The model under review builds one solid part; all positions refer to its coordinate system, in mm. A direction names the side the tool comes from. Round coordinates to 2 decimals unless told otherwise and drop trailing zeros. Write each loop counter-clockwise with the first axis right and the second up, starting at its lowest first coordinate (ties: lowest second). Pieces come first, ordered by that corner, then holes. Notation, with made-up numbers: M 54.5,51.25 L 80.5,51.25 A12 cw 80.5,59.25 Z; hole C 2.5,-26.5 d11. An arc over 180 degrees is marked long. One line per item, written item: value. Start each with the question number.
1) Tool access review of faces 1 (the face through (1, 5, 26.5)), 2 (the face through (-100, 5, 26.5)), 3 (the face through (99.29, -6.52, 3.19)), 4 (the face through (-22, 8, -13.95)): name each direction out of +Z, -Z, +X, -X, +Y, -Y from which nothing blocks a thin tool from reaching the whole face with its end or side.
2) Mouldability with a two-part tool opening along X and no side actions: class faces 5 (the face through (-31, 10, 13)), 6 (the face through (-113.57, 4.93, 25)), 7 (the face through (-41, 3, -21.227)) as +X half, -X half, draft (parallel to the pull), parting line (faces both ways), or undercut.
3) Wall thickness on probe 1 along Z at (x, y) = (75, 8.2); probe 2 along Z at (x, y) = (-12.5, 1.5); probe 3 along X at (y, z) = (5, 20.5): over which ranges is each line inside the solid? List them lowest first.
4) Take a section at B-B, the plane x = 75. Write out the cut boundary in (y, z).
5) Take a section at A-A, the plane x = -5. Write out the cut boundary in (y, z).
6) For P1, Ø1.8, axis at x = -50.5, y = 2.5, coming from the +Z side; P2, Ø8, axis at y = -5, z = 16.5, coming from the -X side; P3, Ø3, axis at x = -52.5, y = 7.5, coming from the -Z side; P4, Ø1.5, axis at x = -71.5, y = -1, coming from the -Z side, all flat-tipped, find the tip position at first contact; note any pin that passes through.
from build123d import *

# Parameters (mm, degrees)
BOSS_EXTRUDE1_DEPTH     = 10
SKETCH2_W               = 50
SKETCH2_H               = 42.5
CUT_EXTRUDE1_DEPTH      = 6
CUT_EXTRUDE7_REACH      = 111.659
SKETCH10_R              = 14.5
CUT_EXTRUDE8_DEPTH      = 110.658560997
CUT_EXTRUDE8_DEPTH_BACK = 3
SKETCH11_R              = 18.75
BOSS_EXTRUDE3_START     = 8
SKETCH12_R              = 30
BOSS_EXTRUDE3_DEPTH     = 8
SKETCH13_R              = 24.5
CUT_EXTRUDE9_DEPTH      = 3
SKETCH14_R              = 18.75
CUT_EXTRUDE10_DEPTH     = 7
CUT_EXTRUDE11_START     = -6
SKETCH15_R              = 24.5
CUT_EXTRUDE11_DEPTH     = 6
CUT_EXTRUDE19_REACH     = 112.095
SKETCH26_W              = 40
SKETCH26_H              = 53
BOSS_EXTRUDE5_DEPTH     = 10
SKETCH19_W              = 46.483409888
SKETCH19_H              = 53
BOSS_EXTRUDE4_DEPTH     = 10
SKETCH23_W              = 7
SKETCH23_H              = 42.47741106
CUT_EXTRUDE18_DEPTH     = 6
FILLET3_R               = 5
SKETCH27_R              = 2.05
SKETCH27_R_2            = 4.962590862
CUT_EXTRUDE20_DEPTH     = 20
CUT_EXTRUDE22_REACH     = 121.269
SKETCH29_R              = 2.05
CUT_EXTRUDE23_REACH     = 121.269
SKETCH30_R              = 1.25


with BuildPart() as part:
    # Sketch1 → Boss-Extrude1 (new body)
    with BuildSketch(Plane(origin=(0, 0, 0), x_dir=(1, 0, 0), z_dir=(0, 1, 0))):
        with BuildLine():
            Line((-52.13627327, 26.5), (60.93763889, 26.5))
            ThreePointArc((60.93763889, 26.5), (105, 0), (60.93763889, -26.5))
            Line((60.93763889, -26.5), (-52.13627327, -26.5))
            Line((-52.13627327, -26.5), (-60.93763889, -26.5))
            ThreePointArc((-60.93763889, -26.5), (-105, 0), (-60.93763889, 26.5))
            Line((-60.93763889, 26.5), (-52.13627327, 26.5))
        make_face()
    extrude(amount=BOSS_EXTRUDE1_DEPTH)

    # Sketch2 → Cut-Extrude1 (cut)
    with BuildSketch(Plane.XZ):
        with Locations((-37.25, 0.02258894)):
            Rectangle(SKETCH2_W, SKETCH2_H)
    extrude(amount=-CUT_EXTRUDE1_DEPTH, mode=Mode.SUBTRACT)

    # Sketch10 → Cut-Extrude7 (cut, up to next)
    with BuildSketch(Plane.XZ, mode=Mode.PRIVATE) as cut_extrude7_sk1:
        with Locations(Location((75, 0, 0), (0, 0, 270))):
            Circle(SKETCH10_R)
    cut_extrude7_tool1 = extrude(cut_extrude7_sk1.sketch, amount=-CUT_EXTRUDE7_REACH, mode=Mode.PRIVATE) & part.part
    add(cut_extrude7_tool1.solids().sort_by_distance((75, 0, 0))[0], mode=Mode.SUBTRACT)

    # Sketch11 → Cut-Extrude8 (cut, two sides: drawn at the far end of the back side and taken through both)
    with BuildSketch(Plane.XZ.offset(-CUT_EXTRUDE8_DEPTH_BACK)):
        with Locations(Location((75, 0, 0), (0, 0, 90))):
            Circle(SKETCH11_R)
    extrude(amount=CUT_EXTRUDE8_DEPTH + CUT_EXTRUDE8_DEPTH_BACK, mode=Mode.SUBTRACT)

    # Sketch12 → Boss-Extrude3 (add)
    with BuildSketch(Plane.XZ.offset(BOSS_EXTRUDE3_START)):
        with Locations(Location((75, 0, 0), (0, 0, 270))):
            Circle(SKETCH12_R)
    extrude(amount=-BOSS_EXTRUDE3_DEPTH)

    # Sketch13 → Cut-Extrude9 (cut)
    with BuildSketch(Plane.XZ.offset(8)):
        with Locations(Location((75, 0, 0), (0, 0, 270))):
            Circle(SKETCH13_R)
    extrude(amount=-CUT_EXTRUDE9_DEPTH, mode=Mode.SUBTRACT)

    # Sketch14 → Cut-Extrude10 (cut)
    with BuildSketch(Plane.XZ.offset(5)):
        with Locations(Location((75, 0, 0), (0, 0, 90))):
            Circle(SKETCH14_R)
    extrude(amount=-CUT_EXTRUDE10_DEPTH, mode=Mode.SUBTRACT)

    # Sketch15 → Cut-Extrude11 (cut)
    with BuildSketch(Plane(origin=(0, 10, 0), x_dir=(1, 0, 0), z_dir=(0, 1, 0)).offset(CUT_EXTRUDE11_START)):
        with Locations(Location((75, 0, 0), (0, 0, 90))):
            Circle(SKETCH15_R)
    extrude(amount=CUT_EXTRUDE11_DEPTH, mode=Mode.SUBTRACT)

    # Sketch25 → Cut-Extrude19 (cut, up to next)
    with BuildSketch(Plane.XZ.offset(-6), mode=Mode.PRIVATE) as cut_extrude19_sk1:
        with BuildLine():
            Line((-33.25, -12), (-41.25, -12))
            ThreePointArc((-41.25, -12), (-53.25, 0), (-41.25, 12))
            Line((-41.25, 12), (-33.25, 12))
            ThreePointArc((-33.25, 12), (-21.25, 0), (-33.25, -12))
        make_face()
    cut_extrude19_tool1 = extrude(cut_extrude19_sk1.sketch, amount=-CUT_EXTRUDE19_REACH, mode=Mode.PRIVATE) & part.part
    # Sketch25 → Cut-Extrude19 (cut, up to next)
    with BuildSketch(Plane.XZ.offset(-6), mode=Mode.PRIVATE) as cut_extrude19_sk2:
        with BuildLine():
            Line((-17.75, -17.05), (-25.75, -17.05))
            ThreePointArc((-25.75, -17.05), (-27.3, -15.5), (-25.75, -13.95))
            Line((-25.75, -13.95), (-17.75, -13.95))
            ThreePointArc((-17.75, -13.95), (-16.2, -15.5), (-17.75, -17.05))
        make_face()
    cut_extrude19_tool2 = extrude(cut_extrude19_sk2.sketch, amount=-CUT_EXTRUDE19_REACH, mode=Mode.PRIVATE) & part.part
    # Sketch25 → Cut-Extrude19 (cut, up to next)
    with BuildSketch(Plane.XZ.offset(-6), mode=Mode.PRIVATE) as cut_extrude19_sk3:
        with BuildLine():
            Line((-48.75, -17.05), (-56.75, -17.05))
            ThreePointArc((-56.75, -17.05), (-58.3, -15.5), (-56.75, -13.95))
            Line((-56.75, -13.95), (-48.75, -13.95))
            ThreePointArc((-48.75, -13.95), (-47.2, -15.5), (-48.75, -17.05))
        make_face()
    cut_extrude19_tool3 = extrude(cut_extrude19_sk3.sketch, amount=-CUT_EXTRUDE19_REACH, mode=Mode.PRIVATE) & part.part
    # Sketch25 → Cut-Extrude19 (cut, up to next)
    with BuildSketch(Plane.XZ.offset(-6), mode=Mode.PRIVATE) as cut_extrude19_sk4:
        with BuildLine():
            Line((-48.75, 13.95), (-56.75, 13.95))
            ThreePointArc((-56.75, 13.95), (-58.3, 15.5), (-56.75, 17.05))
            Line((-56.75, 17.05), (-48.75, 17.05))
            ThreePointArc((-48.75, 17.05), (-47.2, 15.5), (-48.75, 13.95))
        make_face()
    cut_extrude19_tool4 = extrude(cut_extrude19_sk4.sketch, amount=-CUT_EXTRUDE19_REACH, mode=Mode.PRIVATE) & part.part
    # Sketch25 → Cut-Extrude19 (cut, up to next)
    with BuildSketch(Plane.XZ.offset(-6), mode=Mode.PRIVATE) as cut_extrude19_sk5:
        with BuildLine():
            Line((-17.75, 13.95), (-25.75, 13.95))
            ThreePointArc((-25.75, 13.95), (-27.3, 15.5), (-25.75, 17.05))
            Line((-25.75, 17.05), (-17.75, 17.05))
            ThreePointArc((-17.75, 17.05), (-16.2, 15.5), (-17.75, 13.95))
        make_face()
    cut_extrude19_tool5 = extrude(cut_extrude19_sk5.sketch, amount=-CUT_EXTRUDE19_REACH, mode=Mode.PRIVATE) & part.part
    add(cut_extrude19_tool1.solids().sort_by_distance((-37.25, 6, 0))[0], mode=Mode.SUBTRACT)
    add(cut_extrude19_tool2.solids().sort_by_distance((-21.75, 6, -15.5))[0], mode=Mode.SUBTRACT)
    add(cut_extrude19_tool3.solids().sort_by_distance((-52.75, 6, -15.5))[0], mode=Mode.SUBTRACT)
    add(cut_extrude19_tool4.solids().sort_by_distance((-52.75, 6, 15.5))[0], mode=Mode.SUBTRACT)
    add(cut_extrude19_tool5.solids().sort_by_distance((-21.75, 6, 15.5))[0], mode=Mode.SUBTRACT)

    # Sketch26 → Boss-Extrude5 (add)
    with BuildSketch(Plane(origin=(0, 10, 0), x_dir=(1, 0, 0), z_dir=(0, 1, 0))):
        with Locations((-95, 0)):
            Rectangle(SKETCH26_W, SKETCH26_H)
    extrude(amount=-BOSS_EXTRUDE5_DEPTH)

    # Sketch19 → Boss-Extrude4 (add)
    with BuildSketch(Plane(origin=(0, 10, 0), x_dir=(1, 0, 0), z_dir=(0, 1, 0))):
        with Locations((-91.758295056, 0)):
            Rectangle(SKETCH19_W, SKETCH19_H)
    extrude(amount=-BOSS_EXTRUDE4_DEPTH)

    # Sketch23 → Cut-Extrude18 (cut)
    with BuildSketch(Plane.XZ):
        with Locations((-65.75, 0.01129447)):
            Rectangle(SKETCH23_W, SKETCH23_H)
    extrude(amount=-CUT_EXTRUDE18_DEPTH, mode=Mode.SUBTRACT)

    # Fillet3
    fillet3_edges = [part.edges().sort_by_distance(p)[0] for p in [
        (-115, 5, -26.5),
        (-115, 5, 26.5),
    ]]
    fillet(fillet3_edges, radius=FILLET3_R)

    # Sketch27 → Cut-Extrude20 (cut)
    with BuildSketch(Plane(origin=(0, 10, 0), x_dir=(1, 0, 0), z_dir=(0, 1, 0))):
        with Locations(Location((25, -20.5, 0), (0, 0, 270))):
            Circle(SKETCH27_R)
        with Locations(Location((-5, -20.5, 0), (0, 0, 270))):
            Circle(SKETCH27_R)
        with Locations((75, 0)):
            Circle(SKETCH27_R_2)
    cut_extrude20 = extrude(amount=-CUT_EXTRUDE20_DEPTH, mode=Mode.SUBTRACT)

    # Sketch29 → Cut-Extrude22 (cut, up to next)
    with BuildSketch(Plane.XZ, mode=Mode.PRIVATE) as cut_extrude22_sk1:
        with Locations(Location((-109, -15, 0), (0, 0, 270))):
            Circle(SKETCH29_R)
    cut_extrude22_tool1 = extrude(cut_extrude22_sk1.sketch, amount=-CUT_EXTRUDE22_REACH, mode=Mode.PRIVATE) & part.part
    # Sketch29 → Cut-Extrude22 (cut, up to next)
    with BuildSketch(Plane.XZ, mode=Mode.PRIVATE) as cut_extrude22_sk2:
        with Locations(Location((-109, 15, 0), (0, 0, 270))):
            Circle(SKETCH29_R)
    cut_extrude22_tool2 = extrude(cut_extrude22_sk2.sketch, amount=-CUT_EXTRUDE22_REACH, mode=Mode.PRIVATE) & part.part
    add(cut_extrude22_tool1.solids().sort_by_distance((-109, 0, -15))[0], mode=Mode.SUBTRACT)
    add(cut_extrude22_tool2.solids().sort_by_distance((-109, 0, 15))[0], mode=Mode.SUBTRACT)

    # Mirror2: Cut-Extrude20 across plane
    add(cut_extrude20.mirror(Plane.XY), mode=Mode.SUBTRACT)

    # Sketch30 → Cut-Extrude23 (cut, up to next)
    with BuildSketch(Plane.XZ, mode=Mode.PRIVATE) as cut_extrude23_sk1:
        with Locations(Location((24.664028051, 1.845213245, 0), (0, 0, 270))):
            Circle(SKETCH30_R)
    cut_extrude23_tool1 = extrude(cut_extrude23_sk1.sketch, amount=-CUT_EXTRUDE23_REACH, mode=Mode.PRIVATE) & part.part
    # Sketch30 → Cut-Extrude23 (cut, up to next)
    with BuildSketch(Plane.XZ, mode=Mode.PRIVATE) as cut_extrude23_sk2:
        with Locations(Location((33.61486353, -1.337952512, 0), (0, 0, 270))):
            Circle(SKETCH30_R)
    cut_extrude23_tool2 = extrude(cut_extrude23_sk2.sketch, amount=-CUT_EXTRUDE23_REACH, mode=Mode.PRIVATE) & part.part
    add(cut_extrude23_tool1.solids().sort_by_distance((24.664028, 0, 1.845213))[0], mode=Mode.SUBTRACT)
    add(cut_extrude23_tool2.solids().sort_by_distance((33.614864, 0, -1.337953))[0], mode=Mode.SUBTRACT)


solid = part.part
Checked values:
1. face 1: +Z, +Y, -Y
1. face 2: +Z, -X, +Y, -Y
1. face 3: -Y
1. face 4: +Y, -Y
2. face 5: draft
2. face 6: -X half
2. face 7: undercut
3. probe 1: z = -30 to -24.5, 24.5 to 30
3. probe 2: z = -26.5 to -21.23, 21.27 to 26.5
3. probe 3: x = -115 to -69.25, -12.25 to -7.05, -2.95 to 22.95, 27.05 to 61.58, 88.42 to 96.9
4. outline: M -8,-30 L 10,-30 L 10,-24.5 L 4,-24.5 L 4,-14.5 L 3,-14.5 L 3,-18.75 L -5,-18.75 L -5,-24.5 L -8,-24.5 Z; M -8,24.5 L -5,24.5 L -5,18.75 L 3,18.75 L 3,14.5 L 4,14.5 L 4,24.5 L 10,24.5 L 10,30 L -8,30 Z
5. outline: M 0,-26.5 L 10,-26.5 L 10,-22.55 L 0,-22.55 Z; M 0,-18.45 L 10,-18.45 L 10,18.45 L 0,18.45 Z; M 0,22.55 L 10,22.55 L 10,26.5 L 0,26.5 Z
6. P1: stops at z = 26.5
6. P2: stops at x = 47.73
6. P3: stops at z = -26.5
6. P4: passes through
